Autodesk Fusion 360 part; units mm, degrees
sketch "Sketch1" plane through (0, 0, 0) normal (0, 1, 0) x (1, 0, 0)
  line L0 (3, -7.25) -> (-3, -7.25)
  line L1 (-3, -7.25) -> (-3, 7.25)
  line L2 (-3, 7.25) -> (3, 7.25)
  line L3 (3, 7.25) -> (3, -7.25)
  line L4 (3, -7.25) -> (-3, 7.25) construction
  line L5 (-3, -7.25) -> (3, 7.25) construction
  dimension "d1" = 14.5
  dimension "d2" = 6
extrude "Extrude1" add sketch "Sketch1" along normal blind 5
sketch "Sketch2" plane through (0, 0, -7.25) normal (0, 0, -1) x (-1, 0, 0)
  line L0 (-3, 0) -> (3, 0)
  line L1 (3, 0) -> (3, 5)
  line L2 (3, 5) -> (-3, 5)
  line L3 (-3, 5) -> (-3, 0)
  line L4 (-3, 5) -> (3, 0) construction
  circle A0 centre (0, 2.5) radius 2.5
  dimension "d5" = 5
extrude "Extrude2" add sketch "Sketch2" along normal blind 2.5 contours A0
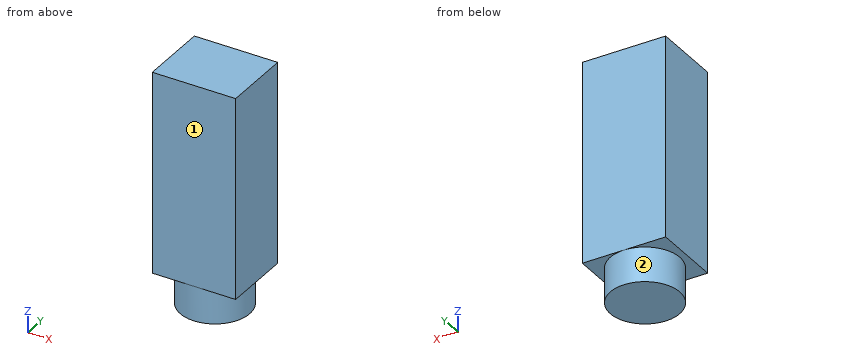
Design review of the part built by this model. Coordinates are the model's own, in mm. Face numbers are marked on the shaded views. A direction names the side the tool comes from. Coordinates: 2 decimals unless noted, no trailing zeros. Order: outer loops, then holes, each group sorted by start corner. A loop starts at its lowest first (then second) coordinate and runs counter-clockwise, first axis right, second up.
Item 1: For the marked faces 1 and 2, list the 3-axis set-ups (+Z, -Z, +X, -X, +Y, -Y) from which the entire face can be reached by the end or side of a thin tool; tool diameter is ignored.
Item 2: For line 1 (Z direction, x = 2.45, y = 1); line 2 (X direction, y = 3, z = -8.75); line 3 (Y direction, x = -1.15, z = -7.5), list the stretches that pass through material, from the lowest coordinate up.
Item 3: Take a section at B-B, the plane x = -2.05. Write out the cut boundary in (y, z).
Item 4: Take a section at A-A, the plane y = 2.5. Write out the cut boundary in (x, z).
The answers:
1. face 1: +Z, -Z, +X, -X, -Y
1. face 2: -Z
2. line 1: z = -7.25 to 7.25
2. line 2: x = -2.45 to 2.45
2. line 3: y = 0.28 to 4.72
3. outline: (0, -7.25) - (1.07, -7.25) - (1.07, -9.75) - (3.93, -9.75) - (3.93, -7.25) - (5, -7.25) - (5, 7.25) - (0, 7.25) - close
4. outline: (-3, -7.25) - (-2.5, -7.25) - (-2.5, -9.75) - (2.5, -9.75) - (2.5, -7.25) - (3, -7.25) - (3, 7.25) - (-3, 7.25) - close
